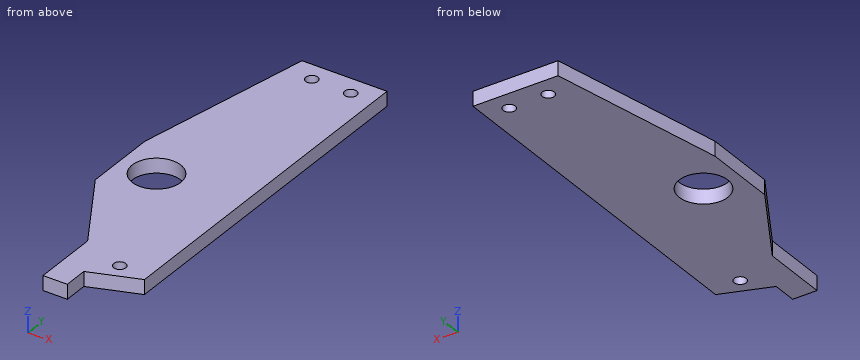
from build123d import *

# Parameters (mm, degrees)
SKETCH1_W           = 10
SKETCH1_H           = 77
BOSS_EXTRUDE1_DEPTH = 3
SKETCH2_W           = 15
SKETCH2_H           = 15
BOSS_EXTRUDE2_DEPTH = 3
BOSS_EXTRUDE3_DEPTH = 3
BOSS_EXTRUDE4_DEPTH = 3
SKETCH5_R           = 5
SKETCH5_R_2         = 1.25
CUT_EXTRUDE1_DEPTH  = 3
CUT_EXTRUDE2_DEPTH  = 10


with BuildPart() as part:
    # Sketch1 → Boss-Extrude1 (new body)
    with BuildSketch(Plane.XY):
        with Locations((-28.110071178, -14.958795526)):
            Rectangle(SKETCH1_W, SKETCH1_H)
    extrude(amount=BOSS_EXTRUDE1_DEPTH)

    # Sketch2 → Boss-Extrude2 (add)
    with BuildSketch(Plane.XY.offset(3)):
        with Locations((-40.610071178, -20.458795526)):
            Rectangle(SKETCH2_W, SKETCH2_H)
    extrude(amount=-BOSS_EXTRUDE2_DEPTH)

    # Sketch3 → Boss-Extrude3 (add)
    with BuildSketch(Plane.XY.offset(3)):
        Polygon((-33.110071178, 23.541204474), (-40.610071178, 23.541204474), (-48.110071178, -12.958795526), (-33.110071178, -12.958795526), align=None)
        Polygon((-48.110071178, -27.958795526), (-33.110071178, -53.458795526), (-33.110071178, -27.958795526), align=None)
    extrude(amount=-BOSS_EXTRUDE3_DEPTH)

    # Sketch4 → Boss-Extrude4 (add)
    with BuildSketch(Plane.XY.offset(3)):
        Polygon((-33.110071178, -53.458795526), (-33.110071178, -58.458795526), (-38.110071178, -58.458795526), (-38.110071178, -44.958795526), align=None)
    extrude(amount=-BOSS_EXTRUDE4_DEPTH)

    # Sketch5 → Cut-Extrude1 (cut)
    with BuildSketch(Plane.XY.offset(3)):
        with Locations((-40.610071178, -20.458795526)):
            Circle(SKETCH5_R)
        with Locations((-29.110071178, -48.458795526)):
            Circle(SKETCH5_R_2)
        with Locations((-35.860071178, 19.541204474)):
            Circle(SKETCH5_R_2)
        with Locations((-27.860071178, 19.541204474)):
            Circle(SKETCH5_R_2)
    extrude(amount=-CUT_EXTRUDE1_DEPTH, mode=Mode.SUBTRACT)

    # Sketch6 → Cut-Extrude2 (cut)
    with BuildSketch(Plane(origin=(0, 0, 0), x_dir=(-1, 0, 0), z_dir=(0, 0, -1))):
        Polygon((23.110071178, -49.817142067), (23.110071178, -53.458795526), (33.110071178, -53.458795526), align=None)
    extrude(amount=-CUT_EXTRUDE2_DEPTH, mode=Mode.SUBTRACT)


solid = part.part
Geometry check sheet. Reference: the model listing, model coordinates, mm. Give positions to 0.01 mm unless a question says otherwise; leave off trailing zeros. Order: outer loops, then holes, each group sorted by start corner. A loop starts at its lowest first (then second) coordinate and runs counter-clockwise, first axis right, second up.
1) Cross-section at D-D (x = -25). Record the boundary of the cut face in (y, z).
Results are:
outline: (-50.51, 0) - (23.54, 0) - (23.54, 3) - (-50.51, 3) - close
2) Gauge pin test, flat ends, axial feed: pin 1 (1.5 mm diameter, centred on y = -57, z = 2, fed in from +X); pin 2 (1.5 mm diameter, centred on y = -10.5, z = 2, fed in from -X); pin 3 (1.5 mm diameter, centred on y = -49, z = 1.5, fed in from -X). Record the tip position at first contact, or that the pin passes through.
Results are:
pin 1: stops at x = -33.11
pin 2: stops at x = -47.76
pin 3: stops at x = -38.11
3) Cross-section at A-A (z = 0.7). Record the boundary of the cut face in (x, y).
Results are:
outline: (-48.11, -27.96) - (-38.11, -44.96) - (-38.11, -58.46) - (-33.11, -58.46) - (-33.11, -53.46) - (-23.11, -49.82) - (-23.11, 23.54) - (-40.61, 23.54) - (-48.11, -12.96) - close; hole circle Ø10 at (-40.61, -20.46); hole circle Ø2.5 at (-35.86, 19.54); hole circle Ø2.5 at (-29.11, -48.46); hole circle Ø2.5 at (-27.86, 19.54)
4) Cross-section at C-C (y = -9). Record the boundary of the cut face in (x, z).
Results are:
outline: (-47.3, 0) - (-23.11, 0) - (-23.11, 3) - (-47.3, 3) - close
5) Cross-section at B-B (x = -41.5). Record the boundary of the cut face in (y, z).
Results are:
outline: (-39.2, 0) - (-25.38, 0) - (-25.38, 3) - (-39.2, 3) - close; (-15.54, 0) - (19.21, 0) - (19.21, 3) - (-15.54, 3) - close
6) Material ranges on probe 1 along Y at (x, z) = (-28.5, 2.25); probe 2 along Y at (x, z) = (-36.25, 1.75); probe 3 along X at (y, z) = (-45.5, 2.7), recorded low to high.
Results are:
probe 1: y = -51.78 to -49.55, -47.37 to 18.47, 20.61 to 23.54
probe 2: y = -58.46 to -22.91, -18.01 to 18.35, 20.73 to 23.54
probe 3: x = -38.11 to -23.11
